Autodesk Inventor part; units mm, degrees
ref_plane "YZ Plane" through (0, 0, 0) normal (1, 0, 0) x (0, 1, 0)
ref_plane "XZ Plane" through (0, 0, 0) normal (0, 1, 0) x (-1, 0, 0)
ref_plane "XY Plane" through (0, 0, 0) normal (0, 0, 1) x (1, 0, 0)
sketch "Sketch1" plane through (0, 0, 0) normal (0, 1, 0) x (-1, 0, 0)
  line L0 (-17, -16) -> (17, -16)
  line L1 (17, -16) -> (17, 16)
  line L2 (17, 16) -> (-17, 16)
  line L3 (-17, 16) -> (-17, -16)
  line L4 (-17, -16) -> (17, 16) construction
  line L5 (17, -16) -> (-17, 16) construction
  point P0 (0, 0)
  dimension "d0" = 32
  dimension "d1" = 34
extrude "Extrusion1" add sketch "Sketch1" along normal blind 2.5
sketch "Sketch2" plane through (0, 2.5, 0) normal (0, 1, 0) x (1, 0, 0)
  line L0 (17, -16) -> (17, 16)
  line L1 (17, -10) -> (-10.85, -10)
  line L2 (-10.85, -10) -> (-10.85, 10)
  line L3 (-10.85, 10) -> (17, 10)
  line L4 (17, 10) -> (17, -10)
  point P0 (0, 0)
  point P1 (17, 10)
  dimension "d4" = 20
  dimension "d5" = 10
  dimension "d6" = 27.85
extrude "Extrusion2" cut sketch "Sketch2" against normal through all
sketch "Sketch3" plane through (0, 2.5, 0) normal (0, 1, 0) x (1, 0, 0)
  line L0 (17, -10) -> (-10.85, -10)
  line L1 (-10.85, -10) -> (-10.85, 10)
  line L2 (-10.85, 10) -> (17, 10)
  line L3 (17, -10) -> (-10.85, -10)
  line L4 (-10.85, -10) -> (-10.85, -9)
  line L5 (-7.35, -9) -> (16, -9)
  line L6 (17, -10) -> (17, -10)
  line L7 (17, 10) -> (-10.85, 10)
  line L8 (-10.85, 10) -> (-10.85, 9)
  line L9 (-7.35, 9) -> (16, 9)
  line L10 (17, 10) -> (17, 10)
  line L11 (-10.85, -10) -> (-8.35, -10)
  line L12 (-8.35, -8) -> (-8.35, 8)
  line L13 (-8.35, 10) -> (-10.85, 10)
  line L14 (-10.85, 10) -> (-10.85, -10)
  arc A0 (17, -10) -> (16, -9) centre (16, -10) ccw
  arc A1 (-8.35, -8) -> (-7.35, -9) centre (-7.35, -8) ccw
  arc A2 (-7.35, 9) -> (-8.35, 8) centre (-7.35, 8) ccw
  arc A3 (16, 9) -> (17, 10) centre (16, 10) ccw
  point P0 (0, 0)
  point P1 (17, -9)
  point P2 (17, 9)
  point P3 (-7.5, -9)
  point P4 (-7.5, 9)
  point P5 (17, 10)
  dimension "d9" = 1
  dimension "d10" = 1
  dimension "d11" = 2.5
  dimension "d14" = 1
extrude "Extrusion3" add sketch "Sketch3" against normal blind 0.4
sketch "Sketch4" plane through (0, 2.5, 0) normal (0, 1, 0) x (1, 0, 0)
  line L0 (-10.85, 10) -> (-10.85, -10)
  line L1 (-17, 16) -> (-17, -16)
  line L2 (-10.85, 10) -> (-10.85, -10)
  line L3 (-10.85, 10) -> (-10.85, -10)
  point P0 (0, 0)
  point P1 (12.55, -13)
  point P2 (-13.95, -13)
  point P3 (-13.95, 13)
  point P4 (12.55, 13)
  point P5 (-13.95, 0)
  point P6 (-1.45, -13)
  point P7 (-1.45, 13)
  dimension "d27" = 13
  dimension "d28" = 13
  dimension "d29" = 12.5
  dimension "d30" = 14
  dimension "d31" = 3.1
hole "Hole1" at (12.55, 2.5, 13) at (-13.95, 2.5, 13) at (-13.95, 2.5, -13) at (12.55, 2.5, -13) at (-1.45, 2.5, 13) at (-1.45, 2.5, -13) at (-13.95, 2.5, 0) direction (0, -1, 0) diameter 2.25 end through all counterbore diameter 3.5 counterbore depth 1.5
fillet "Fillet1" radius 1 6 edges at (-17, 1.25, 16) (-17, 1.25, -16) (17, 1.05, 10) (17, 1.25, 16) (17, 1.05, -10) (17, 1.25, -16)
sketch "Sketch5" plane through (0, 2.5, 0) normal (0, 1, 0) x (1, 0, 0)
  circle A0 centre (12.55, -13) radius 1.75
  line L0 (12.6221, -15.435) -> (8.8746, -15.435)
  line L1 (8.8746, -15.435) -> (8.8746, -12.9967)
  line L2 (8.8746, -12.9967) -> (10.8, -12.9967)
  line L3 (12.6221, -15.435) -> (12.6221, -14.7485)
  point P0 (0, 0)
extrude "Extrusion4" cut sketch "Sketch5" against normal blind 0.5 contours A0 L3 L0 L1 L2
equation "\"d10\" = d9"
properties part number "Flex Circuit Clamp V2"
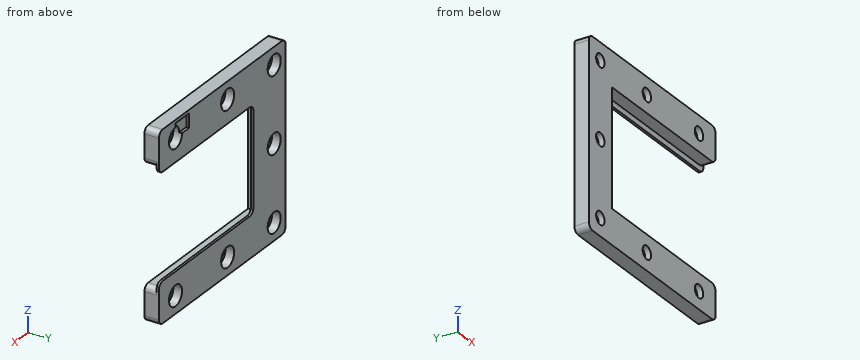
CAD build for the part. Positions are in the model's coordinates, mm. Coordinates: 2 decimals unless noted, no trailing zeros. Order: outer loops, then holes, each group sorted by start corner. A loop starts at its lowest first (then second) coordinate and runs counter-clockwise, first axis right, second up. Notation, with made-up numbers: M 68.25,13 L 95.25,13 A14 ccw 95.25,18 Z; hole C 2,37.5 d3. An arc over 180 degrees is marked long. Answer as CSV lines item,"result".
1) Cut at C-C (y = 1.55). List the corners of the cut face in (x, z), then the cut area to 3 significant figures.
Verdict:
outline,"M -17,-15 A1 ccw -16,-16 L 16,-16 A1 ccw 17,-15 L 17,-11 A1 ccw 16,-10 L -10.85,-10 L -10.85,10 L 16,10 A1 ccw 17,11 L 17,15 A1 ccw 16,16 L -16,16 A1 ccw -17,15 Z; hole C -13.95,-13 d3.5; hole C -13.95,0 d3.5; hole C -13.95,13 d3.5; hole C -1.45,-13 d3.5; hole C -1.45,13 d3.5; hole C 12.55,-13 d3.5; hole C 12.55,13 d3.5"
area,"462 mm2"
2) Drill centre lines: L1, parallel to Z at x = -13.95, y = 1.6; L2, parallel to X at y = 1.9, z = 13; L3, parallel to Z at x = -13.95, y = 0.75 (3 decimals). Where is each one in solid material? Low to high. Write a range as from..to.
Verdict:
L1,"-16..-14.75, -11.25..-1.75, 1.75..11.25, 14.75..16"
L2,"-17..-15.7, -12.2..-3.2, 0.3..10.8, 14.3..17"
L3,"-16..-14.125, -11.875..-1.125, 1.125..11.875, 14.125..16"
3) Cut at A-A (z = 0). List the corners of the cut face in (x, y) (3 decimals).
Verdict:
outline,"M -17,0 L -15.075,0 L -15.075,1 L -15.7,1 L -15.7,2.5 L -17,2.5 Z; M -12.825,0 L -10.85,0 L -10.85,2.1 L -8.35,2.1 L -8.35,2.5 L -12.2,2.5 L -12.2,1 L -12.825,1 Z"
4) Cut at D-D (x = -13.95). List the corners of the cut face in (y, z) (3 decimals).
Verdict:
outline,"M 0,-16 L 2.5,-16 L 2.5,-14.75 L 1,-14.75 L 1,-14.125 L 0,-14.125 Z; M 0,-11.875 L 1,-11.875 L 1,-11.25 L 2.5,-11.25 L 2.5,-1.75 L 1,-1.75 L 1,-1.125 L 0,-1.125 Z; M 0,1.125 L 1,1.125 L 1,1.75 L 2.5,1.75 L 2.5,11.25 L 1,11.25 L 1,11.875 L 0,11.875 Z; M 0,14.125 L 1,14.125 L 1,14.75 L 2.5,14.75 L 2.5,16 L 0,16 Z"
5) Flat gauge pins, fed straight in: P1, Ø2, axis at x = 12.55, z = -13, coming from the -Y side; P2, Ø3, axis at x = -13.95, z = 0, coming from the +Y side. Where does each tip first touch, or does it go through?
Verdict:
P1,"through"
P2,"y = 1"
6) Cut at B-B (x = -6). List the corners of the cut face in (y, z).
Verdict:
outline,"M 0,-16 L 2.5,-16 L 2.5,-9 L 2.1,-9 L 2.1,-10 L 0,-10 Z; M 0,10 L 2.1,10 L 2.1,9 L 2.5,9 L 2.5,16 L 0,16 Z"
